from build123d import *

# Parameters (mm, degrees)
ESQUISSE1_R          = 11
BASE_EXTRUSION_DEPTH = 2
ESQUISSE3_R          = 1.75
BOSS_EXTRU_1_DEPTH   = 13
CHANFREIN1_SIZE      = 0.5
CONG_1_R             = 0.5


with BuildPart() as part:
    # Esquisse1 → Base-Extrusion (new body)
    with BuildSketch(Plane.XY):
        Circle(ESQUISSE1_R)
    extrude(amount=BASE_EXTRUSION_DEPTH)

    # Esquisse3 → Boss.-Extru.1 (add)
    with BuildSketch(Plane.XY.offset(2)):
        with Locations(Location((0, 0, 0), (0, 0, 180))):
            Circle(ESQUISSE3_R)
    extrude(amount=BOSS_EXTRU_1_DEPTH)

    # Chanfrein1
    chanfrein1_edges = [part.edges().sort_by_distance(p)[0] for p in [
        (1.75, 0, 15),
    ]]
    chamfer(chanfrein1_edges, length=CHANFREIN1_SIZE)

    # Congé1
    cong_1_edges = [part.edges().sort_by_distance(p)[0] for p in [
        (1.75, 0, 2),
    ]]
    fillet(cong_1_edges, radius=CONG_1_R)


solid = part.part
Source: CAD feature listing. Evaluate the final solid. Frame: model axes, mm. A direction names the side the tool comes from. Round coordinates to 2 decimals unless told otherwise and drop trailing zeros. Loops run counter-clockwise (first coordinate to the right, second up) from the corner with the lowest first, then second, coordinate; pieces in that order, holes last.
Q1. Section C-C, the plane z = 8. Return loops of the section in (x, y), plus the area to 3 significant figures.
Q2. Section A-A, the plane y = 0. Return loops of the section in (x, z), plus the area to 3 significant figures.
Q3. Access query for faces 1 (the face through (-1.617, 0.67, 8.416)), 2 (the face through (0, 0, 0)). Directions: +Z, -Z, +X, -X, +Y, -Y. A direction counts if a zero-diameter tool reaches every point of the face in a straight line with its end or side. Return the directions, or none.
Q4. Section D-D, the plane x = -7.75. Return loops of the section in (y, z), plus the area to 3 significant figures.
Q5. Ray query, line 1 (Z direction, x = 5, y = 0); line 2 (X direction, y = -8, z = 1.25); line 3 (Z direction, x = 1.75, y = 1). Return the intervals inside material, ascending.
Q6. First-contact query: P1, Ø1.5, axis at y = -8.5, z = 3, coming from the -X side; P2, Ø3, axis at x = -5.5, y = -5, coming from the +Z side; P3, Ø2, axis at x = 2, z = 13.5, coming from the +Y side. Flat tips, straight axial feed; report the tip coordinate or a pass-through.
Solutions:
1. outline: circle Ø3.5 at (0, 0)
1. area: 9.62 mm2
2. outline: (-11, 0) - (11, 0) - (11, 2) - (2.25, 2) arc R0.5 cw to (1.75, 2.5) - (1.75, 14.5) - (1.25, 15) - (-1.25, 15) - (-1.75, 14.5) - (-1.75, 2.5) arc R0.5 cw to (-2.25, 2) - (-11, 2) - close
2. area: 89.4 mm2
3. face 1: +Z
3. face 2: -Z, +X, -X, +Y, -Y
4. outline: (-7.81, 0) - (7.81, 0) - (7.81, 2) - (-7.81, 2) - close
4. area: 31.2 mm2
5. line 1: z = 0 to 2
5. line 2: x = -7.55 to 7.55
5. line 3: z = 0 to 2.06
6. P1: passes through
6. P2: stops at z = 2
6. P3: stops at y = 1.44
